Check sheet for the modelled part. Datum: model origin and axes. Units: mm. Give positions to 0.01 mm unless a question says otherwise; leave off trailing zeros. Write each loop counter-clockwise with the first axis right and the second up, starting at its lowest first coordinate (ties: lowest second). Pieces come first, ordered by that corner, then holes. Notation, with made-up numbers: (12, 59.5) -> (32, 59.5) arc R21 ccw to (32, 87.5) -> close; hole circle Ø11 at (-26, 19.5). An arc over 180 degrees is marked (long way). Use a Markdown table: item, result. Add a question column.
1. Scan lines: probe 1 along Y at (x, z) = (-14, 2); probe 2 along X at (y, z) = (34, 2.75); probe 3 along Y at (x, z) = (-43, 1.4). Record each from-to range of solid material in increasing order. Write a range as [from, to].
2. Cross-section at A-A (x = 17). Enter the section's corners in (y, z), then the cut area to 3 significant figures.
3. Cross-section at C-C (z = 0.75). Count the separate pieces of the cut face and the enclosed holes in it, then the cut area to 3 significant figures.
4. Gauge pin test, flat ends, axial feed: P1, Ø3, axis at x = 13.71, y = 97.29, coming from the -Z side; P2, Ø0.9, axis at x = 38, z = 1.5, coming from the +Y side; P3, Ø0.9, axis at y = -26, z = 1, coming from the -X side; P4, Ø0.9, axis at x = 29, z = 1, coming from the -Y side. Record the tip position at first contact, or that the pin passes through.
5. Cross-section at B-B (y = -7.5). Enter the section's corners in (x, z), then the cut area to 3 significant figures.
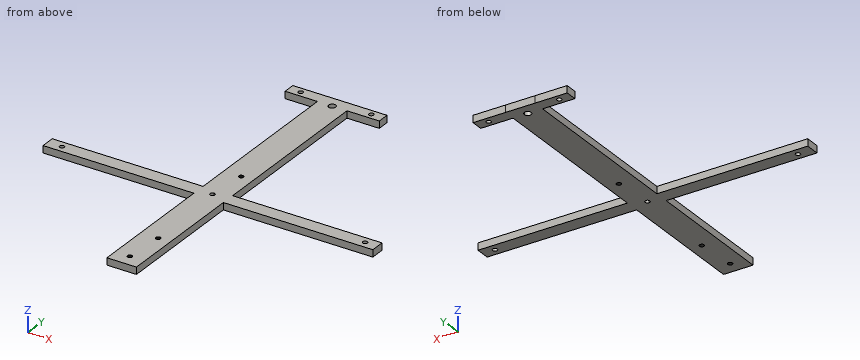
from build123d import *

# Parameters (mm, degrees)
F0_W     = 64.0446986989
F0_H     = 6
F0_R     = 1
F0_W_2   = 63.4251574627
F1_DEPTH = 3


# Not quite as in the source:
# - ends of sketch curves that miss each other by under 0.0002 mm in the source are joined
# - a feature names something its author has since deleted; it is built from what else it names


with BuildPart() as f1:
    # F0 (on Top) → F1 (new body)
    with BuildSketch(Plane.XY):
        Polygon((-7.5510093011, -42.2321148217), (-1.289947, -42.2321148217), (4.9791345373, -42.2321148217), (4.9791345373, 14.358856), (-1.595708, 14.358856), (-7.5510093011, 14.358856), align=None)
        Polygon((-0.297832, -36.78021), (-0.289947, -36.905543), (-0.297832, -37.030876), (-0.321364, -37.154233), (-0.360171, -37.273667), (-0.41364, -37.387296), (-0.48093, -37.493328), (-0.560978, -37.59009), (-0.652523, -37.676056), (-0.75412, -37.749871), (-0.864168, -37.81037), (-0.98093, -37.856599), (-1.102566, -37.88783), (-1.227157, -37.90357), (-1.352738, -37.90357), (-1.477328, -37.88783), (-1.598964, -37.856599), (-1.715726, -37.81037), (-1.825774, -37.749871), (-1.927371, -37.676056), (-2.018916, -37.59009), (-2.098964, -37.493328), (-2.166254, -37.387296), (-2.219724, -37.273667), (-2.25853, -37.154233), (-2.282062, -37.030876), (-2.289947, -36.905543), (-2.282062, -36.78021), (-2.25853, -36.656853), (-2.219724, -36.537418), (-2.166254, -36.423789), (-2.098964, -36.317758), (-2.018916, -36.220996), (-1.927371, -36.13503), (-1.825774, -36.061215), (-1.715726, -36.000716), (-1.598964, -35.954486), (-1.477328, -35.923256), (-1.352738, -35.907516), (-1.227157, -35.907516), (-1.102566, -35.923256), (-0.98093, -35.954486), (-0.864168, -36.000716), (-0.75412, -36.061215), (-0.652523, -36.13503), (-0.560978, -36.220996), (-0.48093, -36.317758), (-0.41364, -36.423789), (-0.360171, -36.537418), (-0.321364, -36.656853), align=None, mode=Mode.SUBTRACT)
        Polygon((0.834477, -20.078598), (0.842362, -20.203931), (0.834477, -20.329264), (0.810945, -20.452621), (0.772138, -20.572056), (0.718669, -20.685685), (0.651379, -20.791716), (0.571331, -20.888478), (0.479786, -20.974444), (0.378189, -21.048259), (0.268141, -21.108758), (0.151379, -21.154988), (0.029743, -21.186218), (-0.094848, -21.201958), (-0.220429, -21.201958), (-0.345019, -21.186218), (-0.466655, -21.154988), (-0.583417, -21.108758), (-0.693465, -21.048259), (-0.795062, -20.974444), (-0.886607, -20.888478), (-0.966655, -20.791716), (-1.033945, -20.685685), (-1.087415, -20.572056), (-1.126221, -20.452621), (-1.149753, -20.329264), (-1.157638, -20.203931), (-1.149753, -20.078598), (-1.126221, -19.955241), (-1.087415, -19.835807), (-1.033945, -19.722178), (-0.966655, -19.616146), (-0.886607, -19.519384), (-0.795062, -19.433418), (-0.693465, -19.359603), (-0.583417, -19.299104), (-0.466655, -19.252875), (-0.345019, -19.221644), (-0.220429, -19.205904), (-0.094848, -19.205904), (0.029743, -19.221644), (0.151379, -19.252875), (0.268141, -19.299104), (0.378189, -19.359603), (0.479786, -19.433418), (0.571331, -19.519384), (0.651379, -19.616146), (0.718669, -19.722178), (0.772138, -19.835807), (0.810945, -19.955241), align=None, mode=Mode.SUBTRACT)
        with Locations((-39.5733586505, 17.358856)):
            Rectangle(F0_W, F0_H)
        with Locations((-65.4838681221, 17.358856)):
            Circle(F0_R, mode=Mode.SUBTRACT)
        with BuildLine():
            Line((-7.5510093011, 20.358856), (-7.5510093011, 14.358856))
            Line((-7.5510093011, 14.358856), (-1.595708, 14.358856))
            Line((-1.595708, 14.358856), (-1.595708, 16.358856))
            ThreePointArc((-1.595708, 16.358856), (-2.595708, 17.358856), (-1.595708, 18.358856))
            Line((-1.595708, 18.358856), (-1.595708, 20.358856))
            Line((-1.595708, 20.358856), (-7.5510093011, 20.358856))
        make_face()
        with BuildLine():
            Line((-1.595708, 14.358856), (4.9791345373, 14.358856))
            Line((4.9791345373, 14.358856), (4.9791345373, 20.358856))
            Line((4.9791345373, 20.358856), (-1.595708, 20.358856))
            Line((-1.595708, 20.358856), (-1.595708, 18.358856))
            ThreePointArc((-1.595708, 18.358856), (-0.8886012188, 18.0659627812), (-0.595708, 17.358856))
            ThreePointArc((-0.595708, 17.358856), (-0.8886012188, 16.6517492188), (-1.595708, 16.358856))
            Line((-1.595708, 16.358856), (-1.595708, 14.358856))
        make_face()
        with Locations((36.6917132686, 17.358856)):
            Rectangle(F0_W_2, F0_H)
        with Locations((63.1569251418, 17.358856)):
            Circle(F0_R, mode=Mode.SUBTRACT)
        Polygon((-7.5510093011, 39.788339287), (-7.5510093011, 20.358856), (-1.595708, 20.358856), (4.9791345373, 20.358856), (4.9791345373, 28.8824737072), (4.9791345373, 39.788339287), (-1.289947, 39.788339287), align=None)
        Polygon((0.834477, 33.921402), (0.842362, 33.796069), (0.834477, 33.670736), (0.810945, 33.547379), (0.772138, 33.427944), (0.718669, 33.314315), (0.651379, 33.208284), (0.571331, 33.111522), (0.479786, 33.025556), (0.378189, 32.951741), (0.268141, 32.891242), (0.151379, 32.845012), (0.029743, 32.813782), (-0.094848, 32.798042), (-0.220429, 32.798042), (-0.345019, 32.813782), (-0.466655, 32.845012), (-0.583417, 32.891242), (-0.693465, 32.951741), (-0.795062, 33.025556), (-0.886607, 33.111522), (-0.966655, 33.208284), (-1.033945, 33.314315), (-1.087415, 33.427944), (-1.126221, 33.547379), (-1.149753, 33.670736), (-1.157638, 33.796069), (-1.149753, 33.921402), (-1.126221, 34.044759), (-1.087415, 34.164193), (-1.033945, 34.277822), (-0.966655, 34.383854), (-0.886607, 34.480616), (-0.795062, 34.566582), (-0.693465, 34.640397), (-0.583417, 34.700896), (-0.466655, 34.747125), (-0.345019, 34.778356), (-0.220429, 34.794096), (-0.094848, 34.794096), (0.029743, 34.778356), (0.151379, 34.747125), (0.268141, 34.700896), (0.378189, 34.640397), (0.479786, 34.566582), (0.571331, 34.480616), (0.651379, 34.383854), (0.718669, 34.277822), (0.772138, 34.164193), (0.810945, 34.044759), align=None, mode=Mode.SUBTRACT)
        with BuildLine():
            Line((-7.5510093011, 94.7883501649), (-7.5510093011, 39.788339287))
            Line((-7.5510093011, 39.788339287), (-1.289947, 39.788339287))
            Line((-1.289947, 39.788339287), (4.9791345373, 39.788339287))
            Line((4.9791345373, 39.788339287), (4.9791345373, 94.7883501649))
            Line((4.9791345373, 94.7883501649), (0.2140626181, 94.7883501649))
            ThreePointArc((0.2140626181, 94.7883501649), (-1.2859428208, 93.2883392871), (-2.7859373819, 94.7883501649))
            Line((-2.7859373819, 94.7883501649), (-7.5510093011, 94.7883501649))
        make_face()
        Polygon((-21.2859819876, 94.7883501649), (-7.5510093011, 94.7883501649), (-7.5510093011, 99.788339287), (-21.2859819876, 99.7883501649), align=None)
        with Locations((-16.2859819876, 97.2883501649)):
            Circle(F0_R, mode=Mode.SUBTRACT)
        with BuildLine():
            Line((-7.5510093011, 99.788339287), (-7.5510093011, 94.7883501649))
            Line((-7.5510093011, 94.7883501649), (-2.7859373819, 94.7883501649))
            ThreePointArc((-2.7859373819, 94.7883501649), (-1.285931943, 96.288339287), (0.2140626181, 94.788339287))
            Line((0.2140626181, 94.788339287), (4.9791345373, 94.7883501649))
            Line((4.9791345373, 94.7883501649), (4.9791345373, 99.788339287))
            Line((4.9791345373, 99.788339287), (-7.5510093011, 99.788339287))
        make_face()
        Polygon((4.9791345373, 99.788339287), (4.9791345373, 94.7883501649), (18.7140180124, 94.7883501649), (18.7140180124, 99.7883501649), align=None)
        with Locations((13.7140180124, 97.2883501649)):
            Circle(F0_R, mode=Mode.SUBTRACT)
    extrude(amount=F1_DEPTH)


solid = f1.part
Worked answers:
| question | item | result |
|---|---|---|
| 1 | probe 1 | y = [14.36, 20.36], [94.79, 99.79] |
| 1 | probe 2 | x = [-7.55, -1.13], [0.82, 4.98] |
| 1 | probe 3 | y = [14.36, 20.36] |
| 2 | outline | (14.36, 0) -> (20.36, 0) -> (20.36, 3) -> (14.36, 3) -> close; (94.79, 0) -> (99.79, 0) -> (99.79, 3) -> (94.79, 3) -> close |
| 2 | area | 33.0 mm² |
| 3 | separate pieces | 1 |
| 3 | enclosed holes | 9 |
| 3 | area | 2,650 mm² |
| 4 | P1 | stops at z = 0 |
| 4 | P2 | stops at y = 20.36 |
| 4 | P3 | stops at x = -7.55 |
| 4 | P4 | stops at y = 14.36 |
| 5 | outline | (-7.55, 0) -> (4.98, 0) -> (4.98, 3) -> (-7.55, 3) -> close |
| 5 | area | 37.6 mm² |
